Work out the finished part from the listing and answer in its coordinate system (mm). A direction names the side the tool comes from. Round coordinates to 2 decimals unless told otherwise and drop trailing zeros. Order: outer loops, then holes, each group sorted by start corner. A loop starts at its lowest first (then second) coordinate and runs counter-clockwise, first axis right, second up. Notation, with made-up numbers: (16, -5.75) -> (36, -5.75) arc R16 cw to (36, -1.75) -> close; hole circle Ø7 at (-24.5, -35.75). An arc over 180 degrees is marked (long way). Use a Markdown table: item, result. Add a question column.
Item 1: For a pull along X with two mould halves and no side action, classify faces 1 (the cylindrical face through (14.284, 6.261, -0.295)), 2 (the cylindrical face through (15.12, 13.45, -11.59)), 3 (the cylindrical face through (10.6, 6.26, 3.34)), 4 (the flat face through (-2.7, 12.7, 14.2)) as +X half, -X half, draft (parallel to the pull), parting line (faces both ways), or undercut.
Item 2: A cutting plane is placed at B-B, the plane z = 0. Determine the outline of the cut face in (x, y), plus the area to 3 significant figures.
Item 3: A cutting plane is placed at A-A, the plane x = 0. Determine the outline of the cut face in (y, z), plus the area to 3 significant figures.
Item 4: A tool of negligible diameter and unlimited length cuts with its end or side. For faces 5 (the flat face through (5, 14.224, 5)), 6 (the cylindrical face through (-14.284, 6.261, 0.295)), 7 (the flat face through (-5, 12.7, -5)), from which of +Z, -Z, +X, -X, +Y, -Y can it reach the whole face along a straight path? Write none if from no direction.
Item 5: Find the intervals of material crossed by L1, parallel to Z at x = 0, y = 13.35; L2, parallel to Z at x = 0, y = 3.75; L3, parallel to Y at x = 15, z = 10, in increasing order. Write a range as [from, to].
Item 6: Flat-ended cylindrical pins translate along their axes: P1, Ø16.5, axis at x = 0, z = 0, coming from the -Y side; P2, Ø6, axis at x = -2, y = 11, coming from the +Z side; P3, Ø5, axis at y = 9, z = -1, coming from the -X side; P4, Ø18, axis at x = -3.5, z = 5, coming from the -Y side. Find the tip coordinate at first contact, or state that the pin passes through.
Item 7: A cutting plane is placed at D-D, the plane x = -4. Determine the outline of the cut face in (y, z), plus the area to 3 significant figures.
from build123d import *

# Parameters (mm, degrees)
F0_R     = 14.2875
F0_R_2   = 11.1125
F1_DEPTH = 12.7
F2_R     = 19.05
F2_R_2   = 1.5875
F2_R_3   = 6.35
F3_DEPTH = 1.524
F4_R     = 1.5875
F5_DEPTH = 25.4


with BuildPart() as f1:
    # F0 (on Front) → F1 (new body)
    with BuildSketch(Plane.XZ):
        Circle(F0_R)
        Circle(F0_R_2, mode=Mode.SUBTRACT)
    extrude(amount=-F1_DEPTH)

    # F2 (on face) → F3 (join)
    with BuildSketch(Plane(origin=(0, 12.7, 0), x_dir=(-1, 0, 0), z_dir=(0, 1, 0))):
        Circle(F2_R)
        with Locations((0, -15.08125)):
            Circle(F2_R_2, mode=Mode.SUBTRACT)
        Circle(F2_R_3, mode=Mode.SUBTRACT)
        with Locations((0, 15.08125)):
            Circle(F2_R_2, mode=Mode.SUBTRACT)
        with BuildLine():
            ThreePointArc((1.336679, 14.224836), (0, 14.2875), (-1.336679, 14.224836))
            ThreePointArc((-1.336679, 14.224836), (0, 13.49375), (1.336679, 14.224836))
        make_face()
        with BuildLine():
            ThreePointArc((1.336679, -14.224836), (0, -14.2875), (-1.336679, -14.224836))
            ThreePointArc((-1.336679, -14.224836), (-0.446194, -16.604755), (1.5875, -15.08125))
            ThreePointArc((1.5875, -15.08125), (1.523505, -14.635056), (1.336679, -14.224836))
        make_face()
        with BuildLine():
            ThreePointArc((1.336679, -14.224836), (0, -13.49375), (-1.336679, -14.224836))
            ThreePointArc((-1.336679, -14.224836), (0, -14.2875), (1.336679, -14.224836))
        make_face()
        with BuildLine():
            ThreePointArc((1.336679, 14.224836), (1.523505, 14.635056), (1.5875, 15.08125))
            ThreePointArc((1.5875, 15.08125), (-0.446194, 16.604755), (-1.336679, 14.224836))
            ThreePointArc((-1.336679, 14.224836), (0, 14.2875), (1.336679, 14.224836))
        make_face()
    extrude(amount=F3_DEPTH)

    # F4 (on face) → F5 (cut)
    with BuildSketch(Plane(origin=(0, 14.224, 0), x_dir=(-1, 0, 0), z_dir=(0, 1, 0))):
        with Locations((0, 15.08125)):
            Circle(F4_R)
        with Locations((0, -15.08125)):
            Circle(F4_R)
    extrude(amount=-F5_DEPTH, mode=Mode.SUBTRACT)


solid = f1.part
Reported:
| question | item | result |
|---|---|---|
| 1 | face 1 | +X half |
| 1 | face 2 | parting line |
| 1 | face 3 | undercut |
| 1 | face 4 | draft |
| 2 | outline | (-19.05, 12.7) -> (-14.29, 12.7) -> (-14.29, 0) -> (-11.11, 0) -> (-11.11, 12.7) -> (-6.35, 12.7) -> (-6.35, 14.22) -> (-19.05, 14.22) -> close; (6.35, 12.7) -> (11.11, 12.7) -> (11.11, 0) -> (14.29, 0) -> (14.29, 12.7) -> (19.05, 12.7) -> (19.05, 14.22) -> (6.35, 14.22) -> close |
| 2 | area | 119 mm² |
| 3 | outline | (0, -13.49) -> (14.22, -13.49) -> (14.22, -6.35) -> (12.7, -6.35) -> (12.7, -11.11) -> (0, -11.11) -> close; (0, 11.11) -> (12.7, 11.11) -> (12.7, 6.35) -> (14.22, 6.35) -> (14.22, 13.49) -> (0, 13.49) -> close; (12.7, -19.05) -> (14.22, -19.05) -> (14.22, -16.67) -> (12.7, -16.67) -> close; (12.7, 16.67) -> (14.22, 16.67) -> (14.22, 19.05) -> (12.7, 19.05) -> close |
| 3 | area | 89.5 mm² |
| 4 | face 5 | +Z, -Z, +X, -X, +Y |
| 4 | face 6 | -X, -Y |
| 4 | face 7 | -Y |
| 5 | L1 | [-19.05, -16.67], [-13.49, -6.35], [6.35, 13.49], [16.67, 19.05] |
| 5 | L2 | [-13.49, -11.11], [11.11, 13.49] |
| 5 | L3 | [12.7, 14.22] |
| 6 | P1 | y = 12.7 |
| 6 | P2 | z = 19.05 |
| 6 | P3 | x = -14.29 |
| 6 | P4 | y = 0 |
| 7 | outline | (0, -13.72) -> (12.7, -13.72) -> (12.7, -18.63) -> (14.22, -18.63) -> (14.22, -4.93) -> (12.7, -4.93) -> (12.7, -10.37) -> (0, -10.37) -> close; (0, 10.37) -> (12.7, 10.37) -> (12.7, 4.93) -> (14.22, 4.93) -> (14.22, 18.63) -> (12.7, 18.63) -> (12.7, 13.72) -> (0, 13.72) -> close |
| 7 | area | 127 mm² |
